Could you check a few things on this drawing? It's one solid part, dimensions in mm from its lowest x, y, z. A direction names the side the tool comes from. Give positions to 0.01 mm unless a question says otherwise; leave off trailing zeros. Order: outer loops, then holes, each group sorted by start corner. A loop starts at its lowest first (then second) coordinate and runs counter-clockwise, first axis right, second up.
Item 1: I want a section at B-B, the plane y = 35. Write out the boundary of the cut face in (x, z), then the cut area to 3 significant figures.
Item 2: I'm going to push flat-ended pins straight in: pin 1 Ø2 at (y, z) = (13, 14) entering from +X; pin 2 Ø3 at (x, z) = (28.5, 19) entering from -Y; pin 3 Ø2 at (y, z) = (23.5, 10) entering from -X. Where does each tip first touch, or does it pass through?
Item 3: Which directions (+Z, -Z, +X, -X, +Y, -Y) give clear straight access to the entire face, cutting with the end or side of a thin tool? Please do the marked faces 5, 6 and 7.
Item 4: I want a section at C-C, the plane x = 35. Write out the boundary of the cut face in (y, z), then the cut area to 3 significant figures.
Item 5: If we mould it in two halves opening along X, with no side actions, what happens to the marked faces 1, 2, 3 and 4? For each: +X half, -X half, draft (parallel to the pull), parting line (faces both ways), or undercut.
Item 6: I want a section at D-D, the plane z = 13. Write out the boundary of the cut face in (x, y).
Item 7: If I drill on line 1 along X through (y, z) = (31.5, 3.75); line 2 along Y through (x, z) = (36, 16.75); line 3 along Y through (x, z) = (63, 15), over which ranges is the centre line in solid material (lowest first)?
Item 8: I want a section at A-A, the plane z = 19.75. Write out the boundary of the cut face in (x, y).
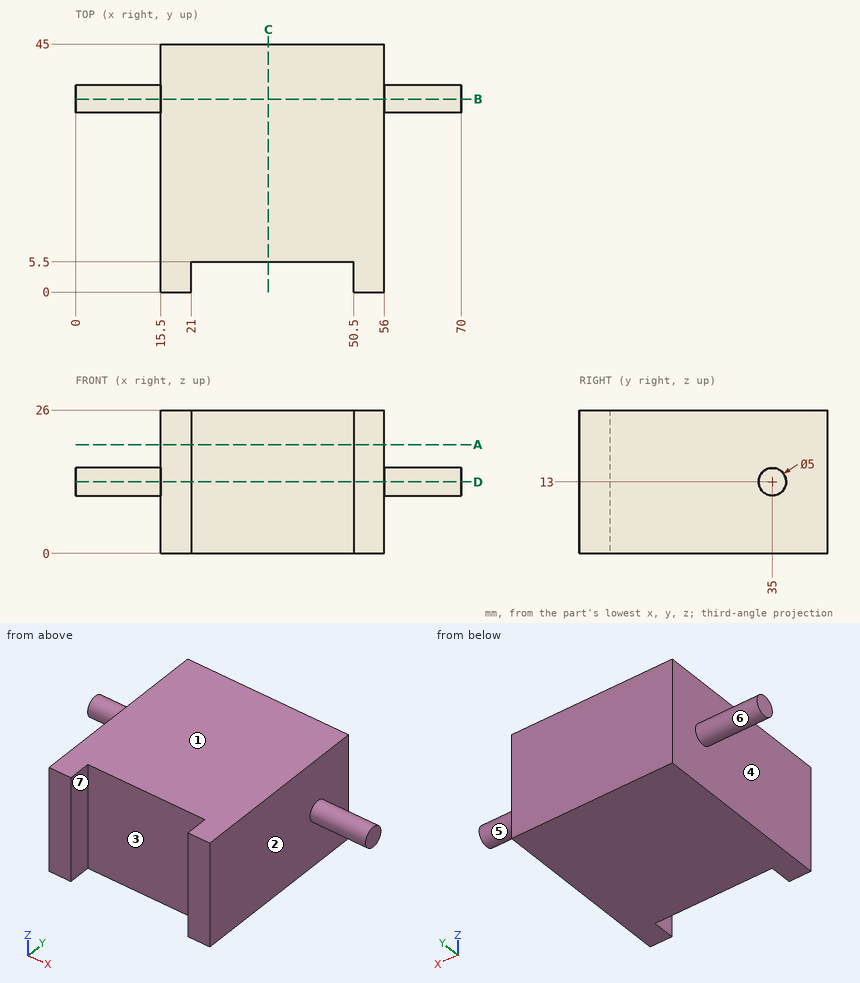
Results list:
1. outline: (0, 10.5) - (15.5, 10.5) - (15.5, 0) - (56, 0) - (56, 10.5) - (70, 10.5) - (70, 15.5) - (56, 15.5) - (56, 26) - (15.5, 26) - (15.5, 15.5) - (0, 15.5) - close
1. area: 1,200 mm2
2. pin 1: stops at x = 56
2. pin 2: stops at y = 5.5
2. pin 3: stops at x = 15.5
3. face 5: +X
3. face 6: -X
3. face 7: +Z, -Z, -Y
4. outline: (5.5, 0) - (45, 0) - (45, 26) - (5.5, 26) - close
4. area: 1,030 mm2
5. face 1: draft
5. face 2: +X half
5. face 3: undercut
5. face 4: -X half
6. outline: (0, 32.5) - (15.5, 32.5) - (15.5, 0) - (21, 0) - (21, 5.5) - (50.5, 5.5) - (50.5, 0) - (56, 0) - (56, 32.5) - (70, 32.5) - (70, 37.5) - (56, 37.5) - (56, 45) - (15.5, 45) - (15.5, 37.5) - (0, 37.5) - close
7. line 1: x = 15.5 to 56
7. line 2: y = 5.5 to 45
7. line 3: y = 33.5 to 36.5
8. outline: (15.5, 0) - (21, 0) - (21, 5.5) - (50.5, 5.5) - (50.5, 0) - (56, 0) - (56, 45) - (15.5, 45) - close
